Design review of the part built by this model. Coordinates are the model's own, in mm. Coordinates: 2 decimals unless noted, no trailing zeros. Write each loop counter-clockwise with the first axis right and the second up, starting at its lowest first coordinate (ties: lowest second). Pieces come first, ordered by that corner, then holes. Notation, with made-up numbers: (2.25, 88) - (7.25, 88) arc R14 cw to (7.25, 109) - close; hole circle Ø3 at (30.25, 32). An arc over 180 degrees is marked (long way). Answer as a JSON object with one key per item and string values.
```python
from build123d import *

# Parameters (mm, degrees)
BOSS_EXTRUDE1_DEPTH      = 9.5
BOSS_EXTRUDE1_DEPTH_BACK = 9.5
SKETCH3_R                = 5
SKETCH3_R_2              = 2.65
CHAMFER1_SIZE            = 0.235
CHAMFER2_SIZE            = 0.3525


with BuildPart() as part:
    # Sketch3 → Boss-Extrude1 (new, two sides: drawn at the far end of the back side and taken through both)
    with BuildSketch(Plane.XY.offset(-BOSS_EXTRUDE1_DEPTH_BACK)):
        Circle(SKETCH3_R)
        Circle(SKETCH3_R_2, mode=Mode.SUBTRACT)
    extrude(amount=BOSS_EXTRUDE1_DEPTH + BOSS_EXTRUDE1_DEPTH_BACK)

    # Chamfer1
    chamfer1_edges = [part.edges().sort_by_distance(p)[0] for p in [
        (-5, 0, -9.5),
        (-5, 0, 9.5),
    ]]
    chamfer(chamfer1_edges, length=CHAMFER1_SIZE)

    # Chamfer2
    chamfer2_edges = [part.edges().sort_by_distance(p)[0] for p in [
        (-2.65, 0, -9.5),
        (-2.65, 0, 9.5),
    ]]
    chamfer(chamfer2_edges, length=CHAMFER2_SIZE)


solid = part.part
```
(1) The part is to be moulded in two halves that separate along Y. For faces 1 (the face through (1, -3, 9.5)), 2 (the face through (-1.08, -4.88, -0.13)), 3 (the face through (2.45, -1.01, -0.13)), say which applies: pulls with the +Y half, pulls with the -Y half, needs draft (parallel to the pull), parting line crosses it, or undercut.
Solved:
{"face 1": "needs draft", "face 2": "parting line crosses it", "face 3": "undercut"}
(2) Take a section at C-C, the plane z = 2.5. Write out the cut boundary in (x, y).
Solved:
{"outline": "circle Ø10 at (0, 0); hole circle Ø5.3 at (0, 0)"}
(3) For pin 1 (3 mm diameter, centred on x = 0, y = 0, fed in from -Z); pin 2 (3 mm diameter, centred on x = 1, z = 3.5, fed in from -Y); pin 3 (5 mm diameter, centred on x = 3, z = 1, fed in from +Y); pin 4 (2 mm diameter, centred on y = 4, z = 1, fed in from -X), all flat-tipped, find the tip position at first contact; note any pin that passes through.
Solved:
{"pin 1": "passes through", "pin 2": "stops at y = -5", "pin 3": "stops at y = 4.97", "pin 4": "stops at x = -4"}
(4) To check wall thickness, follow line 1 (Y direction, x = 0, z = -1.75); line 2 (X direction, y = 4, z = -1); line 3 (Y direction, x = -1, z = 7.5). State the ranges of each line that lie inside material, in increasing order. Write a range as from..to.
Solved:
{"line 1": "y = -5..-2.65, 2.65..5", "line 2": "x = -3..3", "line 3": "y = -4.9..-2.45, 2.45..4.9"}
